The figure shows three views and two pictorial views of one solid part (mm, origin at its lowest corner). Answer the questions. A direction names the side the tool comes from. Round coordinates to 2 decimals unless told otherwise and drop trailing zeros. Loops run counter-clockwise (first coordinate to the right, second up) from the corner with the lowest first, then second, coordinate; pieces in that order, holes last. Notation, with made-up numbers: (56, -11) -> (107, -11) arc R26 cw to (107, 19) -> close; hole circle Ø9 at (-21.75, 20.25). An arc over 180 degrees is marked (long way). Use a Markdown table: item, result. Add a question column.
Q1. For a pull along X with two mould halves and no side action, classify the marked faces 4 and 5 as released by +X, released by -X, zero draft, split by the parting line, or undercut.
Q2. Section B-B on x = 37.5 is taken. Give the vertices of the cut face in (y, z), then the cut area to 3 significant figures.
Q3. Which of the six approach directions +Z, -Z, +X, -X, +Y, -Y give full straight-line access (tool end or side, diameter ignored) to the marked faces 1, 2 and 3?
Q4. Section C-C on x = 80.2 is taken. Give the vertices of the cut face in (y, z).
Q5. Section D-D on y = 11.75 is taken. Give the number of separate pieces and of enclosed holes in the cut face, then the cut area to 3 significant figures.
Q6. Given pin 1 Ø6.5 at (y, z) = (12, 17.5) entering from +X; pin 2 Ø4.5 at (x, y) = (39, 7) entering from -Z; pin 3 Ø3 at (x, z) = (31.5, 11) entering from +Y; pin 4 Ø6.5 at (x, y) = (124.22, 9.77) entering from +Z, each flat-ended and moving along its own axis, determine where each tip first touches the part or whether it passes through.
Q7. Consider line 1 (X direction, y = 1.15, z = 15.5); line 2 (X direction, y = 10, z = 15) (1 decimal); line 3 (X direction, y = 12.5, z = 16.5) (1 decimal). Determine where each line is inside the solid, lowest interval first.
Q8. Section A-A on z = 15.5 is taken. Give the vertices of the cut face in (x, y), then the cut area to 3 significant figures.
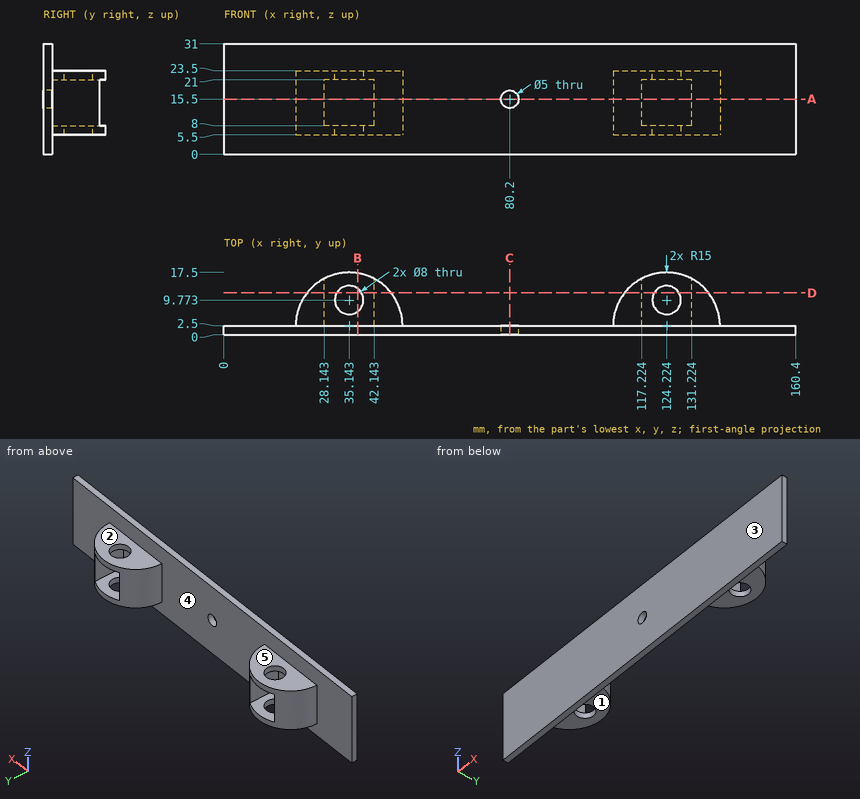
Checked values:
| question | item | result |
|---|---|---|
| 1 | face 4 | undercut |
| 1 | face 5 | zero draft |
| 2 | outline | (0, 0) -> (2.5, 0) -> (2.5, 5.5) -> (6.54, 5.5) -> (6.54, 8) -> (2.5, 8) -> (2.5, 21) -> (6.54, 21) -> (6.54, 23.5) -> (2.5, 23.5) -> (2.5, 31) -> (0, 31) -> close; (13, 5.5) -> (17.31, 5.5) -> (17.31, 8) -> (13, 8) -> close; (13, 21) -> (17.31, 21) -> (17.31, 23.5) -> (13, 23.5) -> close |
| 2 | area | 119 mm2 |
| 3 | face 1 | -Z, +X, -X, +Y |
| 3 | face 2 | +Z, +X, -X, +Y |
| 3 | face 3 | +Z, -Z, +X, -X, -Y |
| 4 | outline | (0, 0) -> (2.5, 0) -> (2.5, 13) -> (0, 13) -> close; (0, 18) -> (2.5, 18) -> (2.5, 31) -> (0, 31) -> close |
| 5 | separate pieces | 4 |
| 5 | enclosed holes | 0 |
| 5 | area | 417 mm2 |
| 6 | pin 1 | stops at x = 137.86 |
| 6 | pin 2 | stops at z = 5.5 |
| 6 | pin 3 | stops at y = 2.5 |
| 6 | pin 4 | passes through |
| 7 | line 1 | x = 0 to 77.7, 82.7 to 160.4 |
| 7 | line 2 | x = 22.2 to 28.1, 42.1 to 48.1, 111.2 to 117.2, 131.2 to 137.2 |
| 7 | line 3 | x = 24 to 28.1, 42.1 to 46.3, 113 to 117.2, 131.2 to 135.4 |
| 8 | outline | (0, 0) -> (77.7, 0) -> (77.7, 2.5) -> (50.14, 2.5) arc R15 ccw to (42.14, 15.77) -> (42.14, 2.5) -> (28.14, 2.5) -> (28.14, 15.77) arc R15 ccw to (20.14, 2.5) -> (0, 2.5) -> close; (82.7, 0) -> (160.4, 0) -> (160.4, 2.5) -> (139.22, 2.5) arc R15 ccw to (131.22, 15.77) -> (131.22, 2.5) -> (117.22, 2.5) -> (117.22, 15.77) arc R15 ccw to (109.22, 2.5) -> (82.7, 2.5) -> close |
| 8 | area | 691 mm2 |
